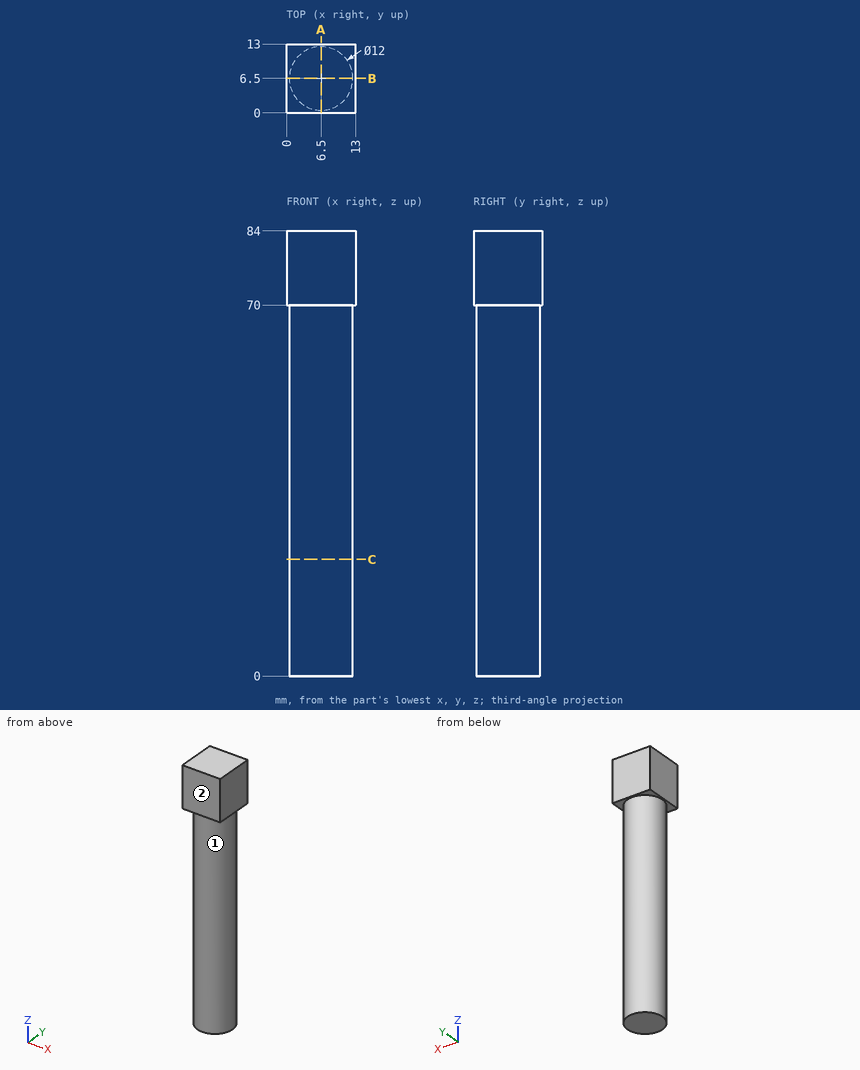
Check sheet for the drawn part. Datum: minimum x, y, z corner. Units: mm. A direction names the side the tool comes from. Round coordinates to 2 decimals unless told otherwise and drop trailing zeros. Order: outer loops, then holes, each group sorted by start corner. A loop starts at its lowest first (then second) coordinate and runs counter-clockwise, first axis right, second up. Notation, with made-up numbers: (-3.5, 26) -> (17.5, 26) arc R13 cw to (17.5, 42) -> close; hole circle Ø8 at (-12, -23). An arc over 180 degrees is marked (long way). Return JSON: item names as keys, results as strings. Group by question number.
Q1. Section check A-A, the plane x = 6.5. Record the boundary of the cut face in (y, z), plus the area to 3 significant figures.
Q2. Section check C-C, the plane z = 22. Record the boundary of the cut face in (x, y), plus the area to 3 significant figures.
Q3. Material ranges on probe 1 along Z at (x, y) = (3.5, 1.25); probe 2 along Y at (x, z) = (6.25, 62); probe 3 along X at (y, z) = (8.25, 62.5), recorded low to high. Write a range as from..to.
Q4. Tool access check on the marked faces 1 and 2. Record the directions out of +Z, -Z, +X, -X, +Y, -Y that give a thin tool (end or side, any length) a straight path to the whole face; none if there is none.
Q5. Gauge pin test, flat ends, axial feed: pin 1 (3 mm diameter, centred on x = 10.5, y = 8.5, fed in from -Z); pin 2 (3 mm diameter, centred on x = 4.5, z = 66.5, fed in from -Y); pin 3 (4 mm diameter, centred on y = 11, z = 25.5, fed in from -X); pin 4 (5 mm diameter, centred on y = 3.5, z = 62.5, fed in from +X). Record the tip position at first contact, or that the pin passes through.
Numbers:
{
 "1": {"outline": "(0, 70) -> (0.5, 70) -> (0.5, 0) -> (12.5, 0) -> (12.5, 70) -> (13, 70) -> (13, 84) -> (0, 84) -> close", "area": "1,020 mm^2"},
 "2": {"outline": "circle Ø12 at (6.5, 6.5)", "area": "113 mm^2"},
 "3": {"probe 1": "70..84", "probe 2": "0.51..12.49", "probe 3": "0.76..12.24"},
 "4": {"face 1": "-Z", "face 2": "+Z, -Z, +X, -X, -Y"},
 "5": {"pin 1": "z = 0", "pin 2": "y = 0.52", "pin 3": "x = 1.05", "pin 4": "x = 12.48"}
}
